Input: part model. Units: mm. Frame: model coordinates. A direction names the side the tool comes from. Coordinates: 2 decimals unless noted, no trailing zeros. Loops run counter-clockwise (first coordinate to the right, second up) from the corner with the lowest first, then second, coordinate; pieces in that order, holes last.
```python
from build123d import *

# Parameters (mm, degrees)
F0_R     = 4
F0_W     = 20
F0_H     = 8
F1_DEPTH = 15
F2_DEPTH = 10
F3_R     = 3.25
F4_DEPTH = 38.001
F5_R     = 8


with BuildPart() as f1:
    # F0 (on Front) → F1 (new body, symmetric)
    with BuildSketch(Plane.XZ):
        Polygon((-20, 0), (0, 0), (0, -30), (15.25, -30), (15.25, 8), (-4.75, 8), (-4.75, 16), (-20, 16), align=None)
        with Locations((-10.75, 8)):
            Circle(F0_R, mode=Mode.SUBTRACT)
        with Locations((5.25, 12)):
            Rectangle(F0_W, F0_H)
    extrude(amount=F1_DEPTH, both=True)

    # F0 (on Front) → F2 (cut, symmetric)
    with BuildSketch(Plane.XZ):
        with Locations((5.25, 12)):
            Rectangle(F0_W, F0_H)
    extrude(amount=F2_DEPTH, both=True, mode=Mode.SUBTRACT)

    # F3 (on face) → F4 (cut, through all)
    with BuildSketch(Plane.XY.offset(8)):
        with Locations((5.25, 0)):
            Circle(F3_R)
    extrude(amount=-F4_DEPTH, mode=Mode.SUBTRACT)

    # F5
    f5_edges = [f1.edges().sort_by_distance(p)[0] for p in [
        (-20, 0, 16),
        (15.25, -12.5, 16),
        (15.25, 12.5, 16),
    ]]
    fillet(f5_edges, radius=F5_R)


solid = f1.part
```
Item 1: Section query C-C (y = -8). Output: boundary loops of the cut face in (x, z), then the cut area to 4 significant figures.
Result:
outline: (-20, 0) - (0, 0) - (0, -30) - (15.25, -30) - (15.25, 8) - (-4.75, 8) - (-4.75, 16) - (-12, 16) arc R8 ccw to (-20, 8) - close; hole circle Ø8 at (-10.75, 8)
area: 797.5 mm2
Item 2: Reachability of faces 4 (the face through (-7, 0, 16)), 5 (the face through (-10, 0, 0)), 6 (the face through (5, -10, 12)) from +Z, -Z, +X, -X, +Y, -Y: full face, straight path, thin tool, end or side. Return the list, or none.
Result:
face 4: +Z, +X, -X, +Y, -Y
face 5: -Z, -X, +Y, -Y
face 6: +Z, +X
Item 3: Mould query, pull axis X, two halves, no side actions, for faces 1 (the face through (12.969, -12.465, 13.594)), 2 (the face through (8.35, 0.98, -10.73)), 3 (the face through (0, 0, -15)). Classes: +X half, -X half, draft (parallel to the pull), parting line (faces both ways), or undercut.
Result:
face 1: +X half
face 2: undercut
face 3: -X half
Item 4: Contact query for flat-ended pins moving along their axis: P1, Ø10, axis at x = -6, y = -4.5, coming from the -Z side; P2, Ø10, axis at x = 4, y = 4, coming from the +Z side; P3, Ø4, axis at y = -5, z = 11.5, coming from the +X side; P4, Ø13, axis at x = -10.75, z = 8, coming from the -Y side. Output: stop coordinate, or through.
Result:
P1: stops at z = 0
P2: stops at z = 8
P3: stops at x = -4.75
P4: stops at y = -15
Item 5: Line query: L1, parallel to Y at x = 5.25, z = -21; L2, parallel to Y at x = -4.5, z = 13; L3, parallel to Z at x = -10.75, y = 0.25. Output: solid intervals per line, ascending.
Result:
L1: y = -15 to -3.25, 3.25 to 15
L2: y = -15 to -10, 10 to 15
L3: z = 0 to 4, 12 to 16
Item 6: Section query A-A (x = 5.25). Output: boundary loops of the cut face in (y, z).
Result:
outline: (-15, -30) - (-3.25, -30) - (-3.25, 8) - (-10, 8) - (-10, 16) - (-15, 16) - close; (3.25, -30) - (15, -30) - (15, 16) - (10, 16) - (10, 8) - (3.25, 8) - close
Item 7: Section query D-D (z = 10.5). Output: boundary loops of the cut face in (x, y).
Result:
outline: (-19.6, -15) - (-13.87, -15) - (-13.87, 15) - (-19.6, 15) - close; (-7.63, -15) - (14.85, -15) - (14.85, -10) - (-4.75, -10) - (-4.75, 10) - (14.85, 10) - (14.85, 15) - (-7.63, 15) - close
Item 8: Section query B-B (y = 0). Output: boundary loops of the cut face in (x, z).
Result:
outline: (-20, 0) - (0, 0) - (0, -30) - (2, -30) - (2, 8) - (-4.75, 8) - (-4.75, 16) - (-12, 16) arc R8 ccw to (-20, 8) - close; (8.5, -30) - (15.25, -30) - (15.25, 8) - (8.5, 8) - close; hole circle Ø8 at (-10.75, 8)
